Can you work these out from the drawing? Everything is in mm from the part's minimum corner. A direction names the side the tool comes from. Round coordinates to 2 decimals unless told otherwise and drop trailing zeros. Write each loop counter-clockwise with the first axis right and the second up, starting at its lowest first coordinate (ties: lowest second). Pieces come first, ordered by that corner, then holes. Notation, with made-up numbers: (21.25, -14.5) -> (42.25, -14.5) arc R27 ccw to (42.25, 5.5) -> close; hole circle Ø11 at (82.5, 88.5). An arc over 180 degrees is marked (long way). Write item = value, one per line. Start each with the question number.
1) I'm going to push flat-ended pins straight in: pin 1 (2 mm diameter, centred on x = 22, y = 17, fed in from +Z); pin 2 (5 mm diameter, centred on x = 13, y = 13, fed in from -Z); pin 3 (1.5 mm diameter, centred on y = 8, z = 9.5, fed in from +X); pin 4 (1.5 mm diameter, centred on x = 6, z = 13, fed in from +Y). Where does each tip first touch, or does it pass through?
2) If I drill on line 1 (Y direction, x = 13, z = 1.45) (1 decimal); line 2 (Y direction, x = 13, z = 11.5), over which ranges is the centre line in solid material (lowest first)?
3) Thinking about a two-plate mould opening in X: for the marked faces 3, 4 and 5, which applies, +X half, -X half, draft (parallel to the pull), parting line (faces both ways), or undercut?
4) Imagine slicing it at C-C, the plane y = 2. Please give me the cut outline in (x, z).
5) Imagine slicing it at D-D, the plane z = 6. Please give me the cut outline in (x, y), then the cut area to 3 significant figures.
6) For the marked faces 1 and 2, which set-ups out of +Z, -Z, +X, -X, +Y, -Y let a thin tool reach every point of the face, with its end or its side?
7) Imagine slicing it at A-A, the plane y = 13. Please give me the cut outline in (x, z) (1 decimal).
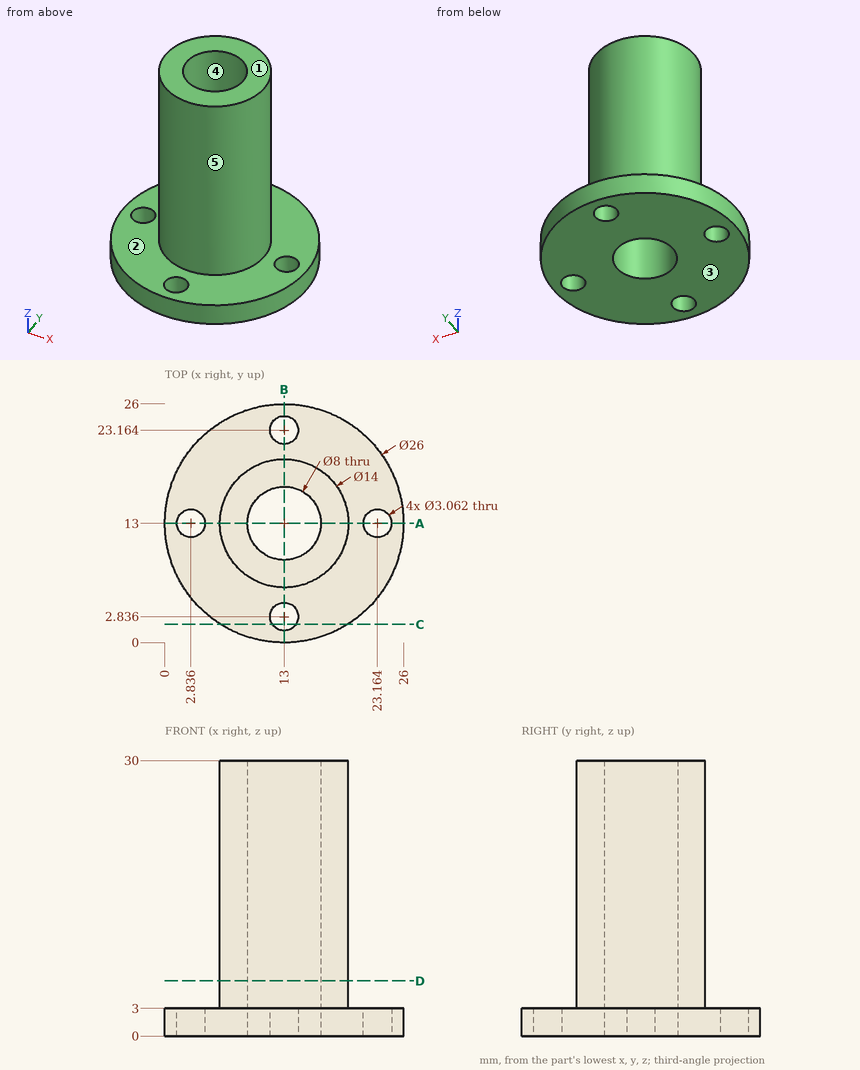
Reported:
q1.pin_1 = 3
q1.pin_2 = through
q1.pin_3 = 18.56
q1.pin_4 = 16.15
q2.line_1 = 0 to 1.3, 4.4 to 9, 17 to 21.6, 24.7 to 26
q2.line_2 = 6 to 9, 17 to 20
q3.face_3 = draft
q3.face_4 = undercut
q3.face_5 = parting line
q4.outline = (6.07, 0) -> (11.72, 0) -> (11.72, 3) -> (6.07, 3) -> close; (14.28, 0) -> (19.93, 0) -> (19.93, 3) -> (14.28, 3) -> close
q5.outline = circle Ø14 at (13, 13); hole circle Ø8 at (13, 13)
q5.area = 104 mm²
q6.face_1 = +Z, +X, -X, +Y, -Y
q6.face_2 = +Z
q7.outline = (0, 0) -> (1.3, 0) -> (1.3, 3) -> (0, 3) -> close; (4.4, 0) -> (9, 0) -> (9, 30) -> (6, 30) -> (6, 3) -> (4.4, 3) -> close; (17, 0) -> (21.6, 0) -> (21.6, 3) -> (20, 3) -> (20, 30) -> (17, 30) -> close; (24.7, 0) -> (26, 0) -> (26, 3) -> (24.7, 3) -> close
